```python
from build123d import *

# Parameters (mm, degrees)
F0_W     = 87
F0_H     = 145
F1_DEPTH = 35
F2_W     = 74
F2_H     = 56
F2_W_2   = 36
F2_H_2   = 31
F2_W_3   = 81
F2_H_3   = 46
F3_DEPTH = 28
F4_D     = 1
F4_DEPTH = 3
F4_START = 28
F4_TIP   = 0.3004303095


with BuildPart() as f1:
    # F0 (on Top) → F1 (new body)
    with BuildSketch(Plane.XY):
        Rectangle(F0_W, F0_H)
    extrude(amount=F1_DEPTH)

    # F2 (on face) → F3 (cut)
    with BuildSketch(Plane.XY.offset(35)):
        with Locations((1.5, 39.5)):
            Rectangle(F2_W, F2_H)
        with Locations((15.5, -6)):
            Rectangle(F2_W_2, F2_H_2)
        with Locations((0, -46.5)):
            Rectangle(F2_W_3, F2_H_3)
    extrude(amount=-F3_DEPTH, mode=Mode.SUBTRACT)

    # F4
    # its depths count from where the whole tool has entered the part; down to there all is cleared
    with Locations(Plane.XY.offset(35)):
        with Locations((-25.5, 62.5)):
            Hole(F4_D / 2, depth=F4_START)
    with Locations(Plane.XY.offset(35).offset(-F4_START)):
        with Locations((-25.5, 62.5)):
            Hole(F4_D / 2, depth=F4_DEPTH)
            with Locations((0, 0, -(F4_DEPTH + F4_TIP / 2))):  # 118° drill point
                Cone(0, F4_D / 2, F4_TIP, mode=Mode.SUBTRACT)


solid = f1.part
```
Geometry check sheet. Reference: the model listing, model coordinates, mm. A direction names the side the tool comes from. Round coordinates to 2 decimals unless told otherwise and drop trailing zeros. Order: outer loops, then holes, each group sorted by start corner. A loop starts at its lowest first (then second) coordinate and runs counter-clockwise, first axis right, second up. Notation, with made-up numbers: (-37, 81.25) - (-19, 81.25) arc R29 ccw to (-19, 109.25) - close; hole circle Ø7 at (64, 40.25). An arc over 180 degrees is marked (long way). Use a Markdown table: item, result. Add a question column.
1) Mould release check, pull along X, two halves, no side actions. Record for faces 1 (the flat face through (15, -6, 7)), 2 (the flat face through (-1, 72.5, 17)), 3 (the flat face through (43.5, -1, 17)): released by +X, released by -X, zero draft, split by the parting line, or undercut.
2) Section check A-A (y = 24.5). Record the cut outline in (x, z), then the cut area to 3 significant figures.
3) Section check C-C (x = 22). Record the cut outline in (y, z).
4) Set-up check for faces 4 (the flat face through (1, 67.5, 21)), 5 (the flat face through (-10, 11, 35)): record each of +Z, -Z, +X, -X, +Y, -Y from which the full face is reachable in a straight line by a thin tool's end or side.
5) Section check D-D (y = 4.5). Record the cut outline in (x, z).
6) Section check B-B (z = 28). Record the cut outline in (x, y), then the cut area to 3 significant figures.
7) Thickness scan on line 1 along Y through (x, z) = (20.5, 18.5); line 2 along Y through (x, z) = (-31, 12.5); line 3 along X through (y, z) = (62.5, 5.8). Record the ranges inside material, lowest first.
8) Gauge pin test, flat ends, axial feed: P1, Ø2, axis at x = 17, y = -35, coming from the +Z side; P2, Ø5, axis at x = -16.5, y = 42, coming from the -Z side. Record the tip position at first contact, or that the pin passes through.
Established:
| question | item | result |
|---|---|---|
| 1 | face 1 | undercut |
| 1 | face 2 | zero draft |
| 1 | face 3 | released by +X |
| 2 | outline | (-43.5, 0) - (43.5, 0) - (43.5, 35) - (38.5, 35) - (38.5, 7) - (-35.5, 7) - (-35.5, 35) - (-43.5, 35) - close |
| 2 | area | 973 mm2 |
| 3 | outline | (-72.5, 0) - (72.5, 0) - (72.5, 35) - (67.5, 35) - (67.5, 7) - (11.5, 7) - (11.5, 35) - (9.5, 35) - (9.5, 7) - (-21.5, 7) - (-21.5, 35) - (-23.5, 35) - (-23.5, 7) - (-69.5, 7) - (-69.5, 35) - (-72.5, 35) - close |
| 4 | face 4 | +Z |
| 4 | face 5 | +Z, +X, -X, +Y, -Y |
| 5 | outline | (-43.5, 0) - (43.5, 0) - (43.5, 35) - (33.5, 35) - (33.5, 7) - (-2.5, 7) - (-2.5, 35) - (-43.5, 35) - close |
| 6 | outline | (-43.5, -72.5) - (43.5, -72.5) - (43.5, 72.5) - (-43.5, 72.5) - close; hole (-40.5, -69.5) - (40.5, -69.5) - (40.5, -23.5) - (-40.5, -23.5) - close; hole (-35.5, 11.5) - (38.5, 11.5) - (38.5, 67.5) - (-35.5, 67.5) - close; hole (-2.5, -21.5) - (33.5, -21.5) - (33.5, 9.5) - (-2.5, 9.5) - close |
| 6 | area | 3,630 mm2 |
| 7 | line 1 | -72.5 to -69.5, -23.5 to -21.5, 9.5 to 11.5, 67.5 to 72.5 |
| 7 | line 2 | -72.5 to -69.5, -23.5 to 11.5, 67.5 to 72.5 |
| 7 | line 3 | -43.5 to -26, -25 to 43.5 |
| 8 | P1 | z = 7 |
| 8 | P2 | z = 0 |
